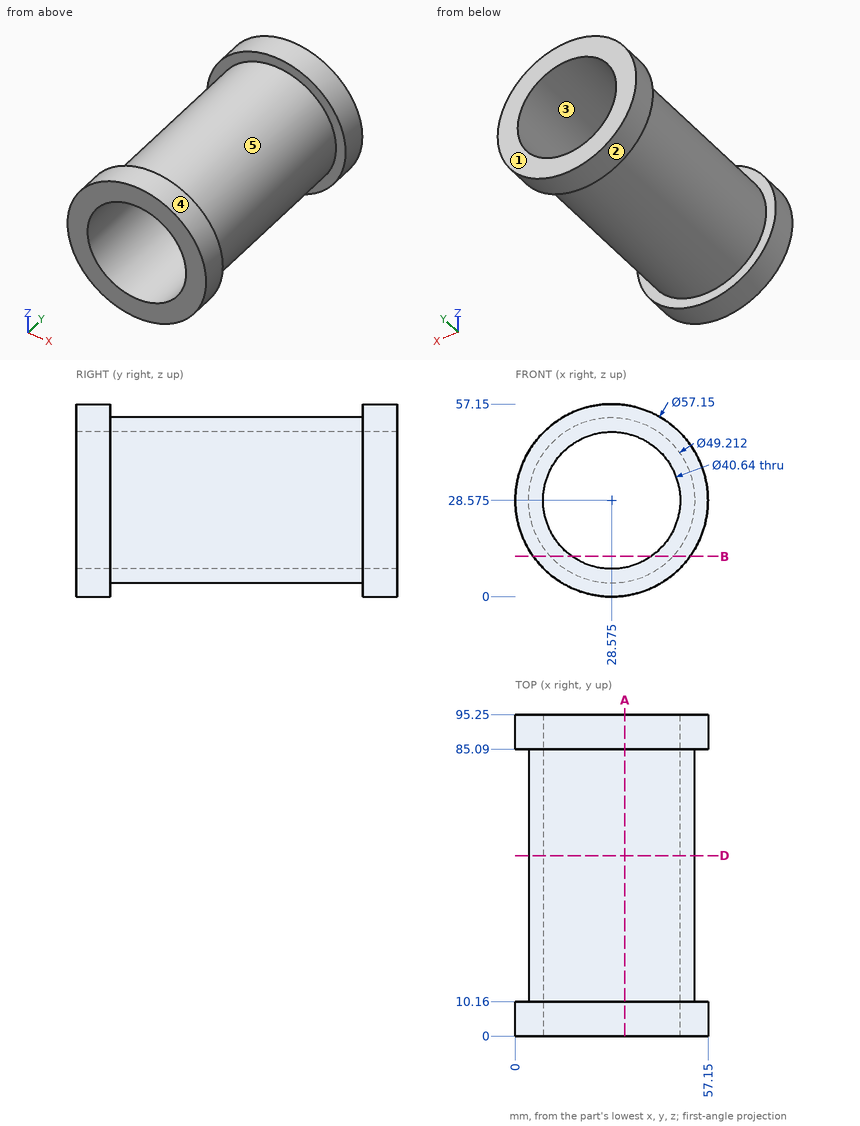
Part print with two shaded views. Sizes in mm from the minimum x, y, z corner. A direction names the side the tool comes from. Round coordinates to 2 decimals unless told otherwise and drop trailing zeros. Loops run counter-clockwise (first coordinate to the right, second up) from the corner with the lowest first, then second, coordinate; pieces in that order, holes last.
1. Two-plate mould, pull along X, no slides. Class the marked faces 1, 2 and 3: pulls with the +X half, pulls with the -X half, needs draft (parallel to the pull), parting line crosses it, or undercut.
Solutions:
face 1: needs draft
face 2: parting line crosses it
face 3: undercut
2. Slice it at A-A (x = 32.5). Give the cut face in (y, z).
Solutions:
outline: (0, 0.27) - (10.16, 0.27) - (10.16, 4.28) - (85.09, 4.28) - (85.09, 0.27) - (95.25, 0.27) - (95.25, 8.64) - (0, 8.64) - close; (0, 48.51) - (95.25, 48.51) - (95.25, 56.88) - (85.09, 56.88) - (85.09, 52.87) - (10.16, 52.87) - (10.16, 56.88) - (0, 56.88) - close
3. Drill centre lines: line 1 along Y through (x, z) = (51.5, 41); line 2 along X through (y, z) = (25, 10) (1 decimal); line 3 along X through (y, z) = (60, 19.5) (1 decimal). Where is each one in solid material? Low to high.
Solutions:
line 1: y = 0 to 10.16, 85.09 to 95.25
line 2: x = 12.4 to 20.3, 36.8 to 44.7
line 3: x = 5.7 to 10.4, 46.8 to 51.4
4. Slice it at D-D (y = 53.5). Give the cut face in (x, z) (1 decimal), and give its area (3 significant figures).
Solutions:
outline: circle Ø49.2 at (28.6, 28.6); hole circle Ø40.6 at (28.6, 28.6)
area: 605 mm2
5. 3-axis set-ups, long thin cutter, end or side, ignore diameter. For the marked faces 4 and 5: which of +Z, -Z, +X, -X, +Y, -Y reach the whole face in a straight line?
Solutions:
face 4: +Y, -Y
face 5: none
6. Slice it at B-B (z = 12). Give the cut face in (x, y), and give its area (3 significant figures).
Solutions:
outline: (5.3, 0) - (16.82, 0) - (16.82, 95.25) - (5.3, 95.25) - (5.3, 85.09) - (10.39, 85.09) - (10.39, 10.16) - (5.3, 10.16) - close; (40.33, 0) - (51.85, 0) - (51.85, 10.16) - (46.76, 10.16) - (46.76, 85.09) - (51.85, 85.09) - (51.85, 95.25) - (40.33, 95.25) - close
area: 1,430 mm2
7. Flat gauge pins, fed straight in: pin 1 (8 mm diameter, centred on x = 37, y = 28.5, fed in from -Z); pin 2 (12 mm diameter, centred on y = 34.5, z = 5.5, fed in from +X); pin 3 (3 mm diameter, centred on y = 77, z = 36.5, fed in from -X). Where does each tip first touch, or does it go through?
Solutions:
pin 1: stops at z = 4.37
pin 2: stops at x = 46.29
pin 3: stops at x = 4.82
